Part model, mm, in its own coordinate system. Face numbers are marked on the shaded views. A direction names the side the tool comes from. Coordinates: 2 decimals unless noted, no trailing zeros. Write each loop counter-clockwise with the first axis right and the second up, starting at its lowest first coordinate (ties: lowest second). Pieces come first, ordered by that corner, then holes. Notation, with made-up numbers: (29.5, 8.5) -> (85.5, 8.5) arc R15 cw to (85.5, 18.5) -> close; hole circle Ø2 at (40, 45). An arc over 180 degrees is marked (long way). Write item = value, one per line. Start each with the question number.
Q1. Band-saw the part on C-C, the plane z = -17. List the corners of the cut face in (x, y).
Q2. Band-saw the part on D-D, the plane x = 6. List the corners of the cut face in (y, z).
Q3. Pin check, flat tips, straight feed: P1, Ø4, axis at y = 12.5, z = 0, coming from the -X side; P2, Ø22.5, axis at y = 0, z = 0, coming from the +X side; P3, Ø4, axis at x = 85.5, z = -12, coming from the +Y side. Stop position of each tip, or through.
Q4. Probe line 1 (Y direction, x = 33.5, z = 0); line 2 (Y direction, x = 85, z = 0); line 3 (X direction, y = -1, z = -11). List the from-to ranges inside material, lowest first.
Q5. Pull direction Y, two halves, no side cores. Call the marked faces 1, 2, 3 and 4: released by +Y, released by -Y, zero draft, split by the parting line, or undercut.
Q6. Tool access for the marked faces 5 and 6: list every direction of +Z, -Z, +X, -X, +Y, -Y with a clear straight run to the whole face (end or side of a thin tool).
Q7. Band-saw the part on B-B, the plane x = 84. List the corners of the cut face in (y, z), plus the area to 3 significant figures.
Q8. Band-saw the part on A-A, the plane y = 0. List the corners of the cut face in (x, z) (3 decimals), plus the area to 3 significant figures.
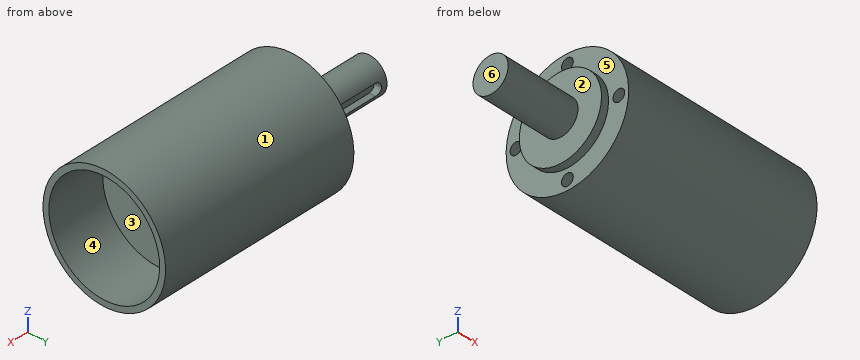
from build123d import *

# Parameters (mm, degrees)
SKETCH1_R          = 5.99
EXTRUDE1_DEPTH     = 25.9
SKETCH2_R          = 13.985
EXTRUDE2_DEPTH     = 2.6
SKETCH3_R          = 20.85
EXTRUDE3_DEPTH     = 69.9
CUT_EXTRUDE1_START = -2
CUT_EXTRUDE1_DEPTH = 20
FILLET8_R          = 2
SKETCH7_R          = 2
CUT_EXTRUDE2_DEPTH = 8
SKETCH9_R          = 18.85
CUT_EXTRUDE3_DEPTH = 20


with BuildPart() as part:
    # Sketch1 → Extrude1 (new body)
    with BuildSketch(Plane(origin=(0, 0, 0), x_dir=(0, 0, -1), z_dir=(1, 0, 0))):
        with Locations(Location((0, 0, 0), (0, 0, 180))):
            Circle(SKETCH1_R)
    extrude(amount=EXTRUDE1_DEPTH)

    # Sketch2 → Extrude2 (add)
    with BuildSketch(Plane(origin=(25.9, 0, 0), x_dir=(0, 0, -1), z_dir=(1, 0, 0))):
        Circle(SKETCH2_R)
    extrude(amount=EXTRUDE2_DEPTH)

    # Sketch3 → Extrude3 (add)
    with BuildSketch(Plane(origin=(28.5, 0, 0), x_dir=(0, 0, -1), z_dir=(1, 0, 0))):
        with Locations(Location((0, 0, 0), (0, 0, 180))):
            Circle(SKETCH3_R)
    extrude(amount=EXTRUDE3_DEPTH)

    # Sketch6 → Cut-Extrude1 (cut)
    with BuildSketch(Plane.ZY.offset(CUT_EXTRUDE1_START)):
        with BuildLine():
            Line((0, 3.49), (0, 5.99))
            ThreePointArc((0, 5.99), (-1.014663299, 5.903436151), (-2, 5.646246541))
            Line((-2, 5.646246541), (-2, 3.49))
            Line((-2, 3.49), (0, 3.49))
        make_face()
        with BuildLine():
            ThreePointArc((2, 5.646246541), (1.014663299, 5.903436151), (0, 5.99))
            Line((0, 5.99), (0, 3.49))
            Line((0, 3.49), (2, 3.49))
            Line((2, 3.49), (2, 5.646246541))
        make_face()
    extrude(amount=-CUT_EXTRUDE1_DEPTH, mode=Mode.SUBTRACT)

    # Fillet8
    fillet8_edges = [part.edges().sort_by_distance(p)[0] for p in [
        (2, 4.56812327, -2),
        (22, 4.56812327, -2),
        (2, 4.56812327, 2),
        (22, 4.56812327, 2),
    ]]
    fillet(fillet8_edges, radius=FILLET8_R - 0.0001)  # a hair under: the kernel refuses the full size

    # Sketch7 → Cut-Extrude2 (cut)
    with BuildSketch(Plane.ZY.offset(-28.5)):
        with Locations((0, 17.5)):
            Circle(SKETCH7_R)
        with Locations((17.5, 0)):
            Circle(SKETCH7_R)
        with Locations((0, -17.5)):
            Circle(SKETCH7_R)
        with Locations((-17.5, 0)):
            Circle(SKETCH7_R)
    extrude(amount=-CUT_EXTRUDE2_DEPTH, mode=Mode.SUBTRACT)

    # Sketch9 → Cut-Extrude3 (cut)
    with BuildSketch(Plane(origin=(98.4, 0, 0), x_dir=(0, 0, -1), z_dir=(1, 0, 0))):
        Circle(SKETCH9_R)
    extrude(amount=-CUT_EXTRUDE3_DEPTH, mode=Mode.SUBTRACT)


solid = part.part
Ans:
q1.outline = (28.5, -12.07) -> (98.4, -12.07) -> (98.4, -8.14) -> (78.4, -8.14) -> (78.4, 8.14) -> (98.4, 8.14) -> (98.4, 12.07) -> (28.5, 12.07) -> (28.5, 1.94) -> (36.5, 1.94) -> (36.5, -1.94) -> (28.5, -1.94) -> close
q2.outline = (3.49, -2) -> (3.49, 2) -> (5.65, 2) arc R5.99 ccw (long way) to (5.65, -2) -> close
q3.P1 = 25.9
q3.P2 = 78.4
q3.P3 = 18.3
q4.line_1 = -20.85 to -19.5, -15.5 to 15.5, 19.5 to 20.85
q4.line_2 = -20.85 to -18.85, 18.85 to 20.85
q4.line_3 = 25.9 to 78.4
q5.face_1 = split by the parting line
q5.face_2 = zero draft
q5.face_3 = undercut
q5.face_4 = undercut
q6.face_5 = -X
q6.face_6 = +Z, -Z, -X, +Y, -Y
q7.outline = circle Ø41.7 at (0, 0); hole circle Ø37.7 at (0, 0)
q7.area = 249 mm2
q8.outline = (0, -5.99) -> (25.9, -5.99) -> (25.9, -13.985) -> (28.5, -13.985) -> (28.5, -15.5) -> (36.5, -15.5) -> (36.5, -19.5) -> (28.5, -19.5) -> (28.5, -20.85) -> (98.4, -20.85) -> (98.4, -18.85) -> (78.4, -18.85) -> (78.4, 18.85) -> (98.4, 18.85) -> (98.4, 20.85) -> (28.5, 20.85) -> (28.5, 19.5) -> (36.5, 19.5) -> (36.5, 15.5) -> (28.5, 15.5) -> (28.5, 13.985) -> (25.9, 13.985) -> (25.9, 5.99) -> (0, 5.99) -> close
q8.area = 2,480 mm2
